Could you check a few things on this model? Use its own coordinates, in mm. A direction names the side the tool comes from. Coordinates: 2 decimals unless noted, no trailing zeros. Write each loop counter-clockwise with the first axis right and the second up, starting at its lowest first coordinate (ties: lowest second). Pieces come first, ordered by that corner, then holes.
```python
from build123d import *

# Parameters (mm, degrees)
F0_R     = 25.4
F0_R_2   = 3.2385
F0_R_3   = 8
F1_DEPTH = 4.7625
F3_DEPTH = 2.38125


with BuildPart() as f1:
    # F0 (on Front) → F1 (new body)
    with BuildSketch(Plane.XZ):
        Circle(F0_R)
        with Locations((0, -16.6624)):
            Circle(F0_R_2, mode=Mode.SUBTRACT)
        Circle(F0_R_3, mode=Mode.SUBTRACT)
        with Locations((-14.430062, 8.3312)):
            Circle(F0_R_2, mode=Mode.SUBTRACT)
        with Locations((14.430062, 8.3312)):
            Circle(F0_R_2, mode=Mode.SUBTRACT)
    extrude(amount=F1_DEPTH)

    # F2 (on face) → F3 (cut)
    with BuildSketch(Plane.XZ.offset(4.7625)):
        with BuildLine():
            ThreePointArc((-3.646079, -10.497322), (-9.623707, -5.55625), (-10.913987, 2.091064))
            ThreePointArc((-10.913987, 2.091064), (-11.409826, 3.527057), (-12.900289, 3.821078))
            ThreePointArc((-12.900289, 3.821078), (-16.190201, 3.905896), (-18.639619, 6.103863))
            ThreePointArc((-18.639619, 6.103863), (-20.156405, 6.905634), (-21.458089, 5.788007))
            ThreePointArc((-21.458089, 5.788007), (-19.247415, -11.1125), (-5.716484, -21.477254))
            ThreePointArc((-5.716484, -21.477254), (-4.097748, -20.908775), (-4.033709, -19.194315))
            ThreePointArc((-4.033709, -19.194315), (-4.712495, -15.974073), (-3.140994, -13.082517))
            ThreePointArc((-3.140994, -13.082517), (-2.650392, -11.644727), (-3.646079, -10.497322))
        make_face()
        with BuildLine():
            ThreePointArc((-7.267908, 8.406258), (0, 11.1125), (7.267908, 8.406258))
            ThreePointArc((7.267908, 8.406258), (8.759433, 8.11767), (9.759295, 9.261439))
            ThreePointArc((9.759295, 9.261439), (11.477705, 12.068177), (14.60591, 13.090452))
            ThreePointArc((14.60591, 13.090452), (16.058657, 14.003141), (15.741606, 15.689247))
            ThreePointArc((15.741606, 15.689247), (0, 22.225), (-15.741606, 15.689247))
            ThreePointArc((-15.741606, 15.689247), (-16.058657, 14.003141), (-14.60591, 13.090452))
            ThreePointArc((-14.60591, 13.090452), (-11.477705, 12.068177), (-9.759295, 9.261439))
            ThreePointArc((-9.759295, 9.261439), (-8.759433, 8.11767), (-7.267908, 8.406258))
        make_face()
        with BuildLine():
            ThreePointArc((10.913987, 2.091064), (9.623707, -5.55625), (3.646079, -10.497322))
            ThreePointArc((3.646079, -10.497322), (2.650392, -11.644727), (3.140994, -13.082517))
            ThreePointArc((3.140994, -13.082517), (4.712495, -15.974073), (4.033709, -19.194315))
            ThreePointArc((4.033709, -19.194315), (4.097748, -20.908775), (5.716484, -21.477254))
            ThreePointArc((5.716484, -21.477254), (19.247415, -11.1125), (21.458089, 5.788007))
            ThreePointArc((21.458089, 5.788007), (20.156405, 6.905634), (18.639619, 6.103863))
            ThreePointArc((18.639619, 6.103863), (16.190201, 3.905896), (12.900289, 3.821078))
            ThreePointArc((12.900289, 3.821078), (11.409826, 3.527057), (10.913987, 2.091064))
        make_face()
    extrude(amount=-F3_DEPTH, mode=Mode.SUBTRACT)


solid = f1.part
```
1. Please list where these lines run through material, in increasing order: line 1 along Z through (x, y) = (0, -1.8); line 2 along X through (y, z) = (-3.4, -12.5); line 3 along X through (y, z) = (-2.9, 2.5).
Verdict:
line 1: z = -25.4 to -19.9, -13.42 to -8, 8 to 25.4
line 2: x = -22.11 to -18.38, -2.73 to 2.73, 18.38 to 22.11
line 3: x = -25.28 to -22.08, -10.89 to -7.6, 7.6 to 10.89, 22.08 to 25.28
2. I want a section at D-D on z = -16. Please give me the cut outline in (x, y).
Verdict:
outline: (-19.73, -4.76) - (-15.43, -4.76) - (-15.43, -2.38) - (-4.72, -2.38) - (-4.72, -4.76) - (-3.17, -4.76) - (-3.17, 0) - (-19.73, 0) - close; (3.17, -4.76) - (4.72, -4.76) - (4.72, -2.38) - (15.43, -2.38) - (15.43, -4.76) - (19.73, -4.76) - (19.73, 0) - (3.17, 0) - close
3. If we mould it in two halves opening along Z, with no side actions, what happens to faces 1 (the face through (-11.39, -3.59, 3.51)), 2 (the face through (-6, 0, 6)), 3 (the face through (-4.72, -3.59, -16.02))? For each: pulls with the +Z half, pulls with the -Z half, needs draft (parallel to the pull), parting line crosses it, or undercut.
Verdict:
face 1: undercut
face 2: needs draft
face 3: undercut
4. I want a section at A-A on z = 0. Please give me the cut outline in (x, y) (1 decimal), plus the area to 3 significant figures.
Verdict:
outline: (-25.4, -4.8) - (-22.2, -4.8) - (-22.2, -2.4) - (-11.1, -2.4) - (-11.1, -4.8) - (-8, -4.8) - (-8, 0) - (-25.4, 0) - close; (8, -4.8) - (11.1, -4.8) - (11.1, -2.4) - (22.2, -2.4) - (22.2, -4.8) - (25.4, -4.8) - (25.4, 0) - (8, 0) - close
area: 113 mm2
5. I want a section at C-C on y = -1.1. Please give me the cut outline in (x, z), plus the area to 3 significant figures.
Verdict:
outline: circle Ø50.8 at (0, 0); hole circle Ø6.48 at (-14.43, 8.33); hole circle Ø16 at (0, 0); hole circle Ø6.48 at (0, -16.66); hole circle Ø6.48 at (14.43, 8.33)
area: 1,730 mm2
6. I want a section at B-B on x = 0. Please give me the cut outline in (y, z) (1 decimal).
Verdict:
outline: (-4.8, -25.4) - (0, -25.4) - (0, -19.9) - (-4.8, -19.9) - close; (-4.8, -13.4) - (0, -13.4) - (0, -8) - (-4.8, -8) - close; (-4.8, 8) - (0, 8) - (0, 25.4) - (-4.8, 25.4) - (-4.8, 22.2) - (-2.4, 22.2) - (-2.4, 11.1) - (-4.8, 11.1) - close
7. On a 3-axis mill with a long thin cutter (end or side, diameter ignored), from which of +Z, -Z, +X, -X, +Y, -Y can I reach the whole of each face in a straight line? I mean faces 4 (the face through (-1.73, -2.35, -7.81)), 5 (the face through (9.68, -3.59, -5.46)). Say none if no direction works.
Verdict:
face 4: +Y, -Y
face 5: -Y
8. For pin 1 (1 mm diameter, centred on x = -7.5, y = -3, fed in from -Z); pin 2 (7.5 mm diameter, centred on x = -14.43, z = 8.33, fed in from +Y); pin 3 (7 mm diameter, centred on x = -4.5, z = 18, fed in from -Y); pin 4 (1 mm diameter, centred on y = -3, z = -16, fed in from -X), each with a flat end and sliding along its axis, tell me the tip position at first contact or that it passes through.
Verdict:
pin 1: stops at z = -24.42
pin 2: stops at y = 0
pin 3: stops at y = -2.38
pin 4: stops at x = -20.12
